Input: part model. Units: mm. Frame: model coordinates. Face numbers are marked on the shaded views. A direction names the side the tool comes from. Coordinates: 2 decimals unless noted, no trailing zeros. Write each loop counter-clockwise with the first axis right and the second up, starting at its lowest first coordinate (ties: lowest second). Pieces come first, ordered by that corner, then holes. Notation, with made-up numbers: M 13,74 L 28,74 A23 ccw 28,96 Z; hole C -28.5,16 d6. An arc over 180 degrees is marked long. Use one line per item in the form item = value.
from build123d import *

# Parameters (mm, degrees)
BOSS_EXTRUDE1_DEPTH   = 5.45
BOSS_EXTRUDE1_2_DEPTH = 5.45
BOSS_EXTRUDE2_DEPTH   = 5.75
BOSS_EXTRUDE3_DEPTH   = 6.001690088
FILLET1_R             = 3.175
SKETCH3_W             = 34.925
SKETCH3_H             = 8
CUT_EXTRUDE1_DEPTH    = 28.618228517
BOSS_EXTRUDE5_DEPTH   = 3.75
FILLET2_R             = 1.778


with BuildPart() as part:
    # Sketch1 → Boss-Extrude1 (new, symmetric)
    with BuildSketch(Plane.XY):
        with BuildLine():
            ThreePointArc((20.625, 0.15), (20.842969199, -0.656220109), (21.43748858, -1.242776279))
            ThreePointArc((21.43748858, -1.242776279), (23.824989974, 0.155664255), (21.42764708, 1.537165571))
            ThreePointArc((21.42764708, 1.537165571), (20.840123711, 0.951322447), (20.625, 0.15))
        make_face()
    extrude(amount=BOSS_EXTRUDE1_DEPTH, both=True)

    # Sketch1<4> → Boss-Extrude2 (add, symmetric)
    with BuildSketch(Plane.XY):
        with BuildLine():
            ThreePointArc((20.625, 0.15), (20.842969199, -0.656220109), (21.43748858, -1.242776279))
            ThreePointArc((21.43748858, -1.242776279), (23.824989974, 0.155664255), (21.42764708, 1.537165571))
            ThreePointArc((21.42764708, 1.537165571), (20.840123711, 0.951322447), (20.625, 0.15))
        make_face()
    extrude(amount=BOSS_EXTRUDE2_DEPTH, both=True)



with BuildPart() as body_2:
    # Sketch1 → Boss-Extrude1 2 (new, symmetric)
    with BuildSketch(Plane.XY):
        with BuildLine():
            Line((-24.525, -3.647655774), (18.025, -3.647655774))
            Line((18.025, -3.647655774), (18.025, 2.354034313))
            Line((18.025, 2.354034313), (-18.725, 2.354034313))
            Line((-18.725, 2.354034313), (-20.4, 2.354034313))
            ThreePointArc((-20.4, 2.354034313), (-20.753553391, 2.207587704), (-20.9, 1.854034313))
            Line((-20.9, 1.854034313), (-20.9, 1.734034313))
            ThreePointArc((-20.9, 1.734034313), (-20.842506971, 1.257939085), (-20.673333333, 0.809216013))
            ThreePointArc((-20.673333333, 0.809216013), (-22.225, -1.75), (-23.776666667, 0.809216013))
            ThreePointArc((-23.776666667, 0.809216013), (-23.607493029, 1.257939085), (-23.55, 1.734034313))
            Line((-23.55, 1.734034313), (-23.55, 1.854034313))
            ThreePointArc((-23.55, 1.854034313), (-23.696446609, 2.207587704), (-24.05, 2.354034313))
            Line((-24.05, 2.354034313), (-24.409724637, 2.354034313))
            ThreePointArc((-24.409724637, 2.354034313), (-24.974960254, 2.154397574), (-25.289436326, 1.644053639))
            ThreePointArc((-25.289436326, 1.644053639), (-25.345434425, 1.158547963), (-25.305905598, 0.671424755))
            Line((-25.305905598, 0.671424755), (-24.525, -3.647655774))
        make_face()
    extrude(amount=BOSS_EXTRUDE1_2_DEPTH, both=True)


with BuildPart() as part_1:
    add(part.part)

    add(body_2.part)  # Boss-Extrude3 merges body 2
    # Sketch2 → Boss-Extrude3 (add)
    with BuildSketch(Plane(origin=(0, -3.647655774, 0), x_dir=(-1, 0, 0), z_dir=(0, -1, 0))):
        Polygon((18.175, 5.45), (-18.025, 5.45), (18.175, 0), align=None)
        Polygon((-25.825, 7.75), (-25.825, 5.75), (-20.01766055, 5.75), (-18.025, 5.45), (18.175, 5.45), (-20.01766055, 7.75), align=None)
        Polygon((18.175, -5.45), (18.175, 0), (-18.025, -5.45), align=None)
        Polygon((-20.01766055, -7.75), (18.175, -5.45), (-18.025, -5.45), (-20.01766055, -5.75), (-25.825, -5.75), (-25.825, -7.75), align=None)
    extrude(amount=-BOSS_EXTRUDE3_DEPTH)

    # Fillet1
    # the kernel refuses this fillet: 3.175 mm, written as the material it takes off along each edge
    with BuildSketch(Plane(origin=(25.825, 2.354034313, -15.687500001), x_dir=(-1, 0, 0), z_dir=(0, 0, 1)), Plane(origin=(25.825, 2.354034313, -2.187500001), x_dir=(-1, 0, 0), z_dir=(0, 0, 1))) as fillet1_piece_1:
        with BuildLine():
            CenterArc((FILLET1_R, FILLET1_R), FILLET1_R, 180, 90)
            Line((0, FILLET1_R), (0, 0))
            Line((0, 0), (FILLET1_R, 0))
        make_face()
    extrude(amount=17.875000002, mode=Mode.SUBTRACT)
    with BuildSketch(Plane(origin=(25.825, -3.647655774, -15.6875), x_dir=(-1, 0, 0), z_dir=(0, 0, 1))) as fillet1_piece_2:
        with BuildLine():
            CenterArc((FILLET1_R, -FILLET1_R), FILLET1_R, 90, 90)
            Line((0, -FILLET1_R), (0, 0))
            Line((0, 0), (FILLET1_R, 0))
        make_face()
    extrude(amount=17.875, mode=Mode.SUBTRACT)
    with BuildSketch(Plane(origin=(25.825, -3.647655774, -2.1875), x_dir=(0, 1, 0), z_dir=(0, 0, 1))) as fillet1_piece_3:
        with BuildLine():
            CenterArc((FILLET1_R, FILLET1_R), FILLET1_R, 180, 90)
            Line((0, FILLET1_R), (0, 0))
            Line((0, 0), (FILLET1_R, 0))
        make_face()
    extrude(amount=17.875, mode=Mode.SUBTRACT)

    # Sketch3 → Cut-Extrude1 (cut, through all)
    with BuildSketch(Plane(origin=(0, -3.647655774, 0), x_dir=(-1, 0, 0), z_dir=(0, -1, 0))):
        with Locations((1.4375, 0)):
            Rectangle(SKETCH3_W, SKETCH3_H)
    extrude(amount=-CUT_EXTRUDE1_DEPTH, mode=Mode.SUBTRACT)

    # Sketch4 → Boss-Extrude5 (add, symmetric)
    with BuildSketch(Plane.XY):
        Polygon((-18.9, -3.647655774), (-20.231157594, -29.047655774), (-24.525, -29.047655774), (-24.525, -3.647655774), align=None)
    extrude(amount=BOSS_EXTRUDE5_DEPTH, both=True)

    # Fillet2
    fillet2_edges = [part_1.edges().sort_by_distance(p)[0] for p in [
        (-24.525, -29.047655774, 0),
        (-20.231157594, -29.047655774, 0),
    ]]
    fillet(fillet2_edges, radius=FILLET2_R)


solid = part_1.part
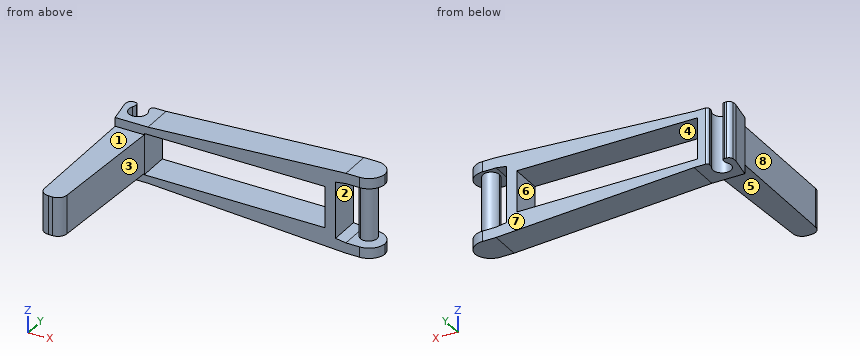
(1) Line query: probe 1 along Y at (x, z) = (-17, -4.5); probe 2 along X at (y, z) = (0, 1.75) (1 decimal); probe 3 along Z at (x, y) = (-22, -9.5). Output: solid intervals per line, ascending.
Computed:
probe_1 = -3.65 to 2.35
probe_2 = -25.2 to -24, -20.5 to -18.9, 16 to 18, 20.6 to 23.8
probe_3 = -3.75 to 3.75
(2) Section query C-C on x = -8. Return the cut outline in (y, z), plus the area to 3 significant figures.
Computed:
outline = M -3.65,-6.06 L 2.35,-6.06 L 2.35,-4 L -3.65,-4 Z; M -3.65,4 L 2.35,4 L 2.35,6.06 L -3.65,6.06 Z
area = 24.8 mm^2
(3) Set-up query: the marked faces 5, 6, 7 and 8. Return all of +Z, -Z, +X, -X, +Y, -Y with unobstructed straight access to the full face (end or side cutting, diameter ignored); none if empty.
Computed:
face_5 = -Z, +X, -X, -Y
face_6 = +Y, -Y
face_7 = +Z, -Z, +X, -X, +Y
face_8 = +Z, -Z, -X, -Y
(4) First-contact query: pin 1 Ø8 at (y, z) = (-17, 0.5) entering from -X (3 decimals); pin 2 Ø5 at (y, z) = (1, 1) entering from +X (3 decimals); pin 3 Ø3 at (x, y) = (-8.5, -0.5) entering from +Z. Flat tips, straight axial feed; report the tip coordinate or a pass-through.
Computed:
pin_1 = -24.525
pin_2 = 23.825
pin_3 = 6.12
(5) Pull-direction query (Z, two-part tool) for the marked faces 1, 2, 3 and 4; classes: pulls with the +Z half, pulls with the -Z half, needs draft (parallel to the pull), parting line crosses it, or undercut.
Computed:
face_1 = pulls with the +Z half
face_2 = undercut
face_3 = needs draft
face_4 = undercut
(6) Section query D-D on x = 6.5. Return the cut outline in (y, z).
Computed:
outline = M -3.65,-6.94 L 2.35,-6.94 L 2.35,-4 L -3.65,-4 Z; M -3.65,4 L 2.35,4 L 2.35,6.94 L -3.65,6.94 Z
(7) Section query A-A on z = 0. Return the cut outline in (x, y) (3 decimals), plus the area to 3 significant figures.
Computed:
outline = M -25.306,0.671 L -24.525,-3.648 L -24.525,-27.27 A1.778 ccw -22.747,-29.048 L -21.918,-29.048 A1.778 ccw -20.143,-27.363 L -18.9,-3.648 L -18.9,2.354 L -20.4,2.354 A0.5 ccw -20.9,1.854 L -20.9,1.734 A2 ccw -20.673,0.809 A1.75 cw long -23.777,0.809 A2 ccw -23.55,1.734 L -23.55,1.854 A0.5 ccw -24.05,2.354 L -24.41,2.354 A0.9 ccw -25.289,1.644 A2.5 ccw Z; M 16.025,-3.648 L 18.025,-3.648 L 18.025,2.354 L 16.025,2.354 Z; C 22.225,0.15 d3.2
area = 169 mm^2
(8) Section query B-B on z = 4.5. Return the cut outline in (x, y) (3 decimals), plus the area to 3 significant figures.
Computed:
outline = M -25.306,0.671 L -24.525,-3.648 L 18.025,-3.648 L 18.025,2.354 L -20.4,2.354 A0.5 ccw -20.9,1.854 L -20.9,1.734 A2 ccw -20.673,0.809 A1.75 cw long -23.777,0.809 A2 ccw -23.55,1.734 L -23.55,1.854 A0.5 ccw -24.05,2.354 L -24.41,2.354 A0.9 ccw -25.289,1.644 A2.5 ccw Z; C 22.225,0.15 d3.2
area = 254 mm^2
